Can you work these out from the model? Positions are in its coordinate system, mm. A direction names the side the tool comes from. Coordinates: 2 decimals unless noted, no trailing zeros. Order: outer loops, then holes, each group sorted by start corner. A loop starts at its lowest first (then second) coordinate and runs counter-clockwise, first axis right, second up. Notation, with made-up numbers: (-39.5, -28.75) -> (-3.5, -28.75) arc R31 cw to (-3.5, 10.25) -> close; hole circle Ø10 at (81, -0.75). An arc over 180 degrees is marked (long way). Write item = value, one per line.
```python
from build123d import *

# Parameters (mm, degrees)
BOSS_EXTRUDE1_DEPTH = 3
SKETCH3_OUTSIDE_W   = 181.071
SKETCH3_OUTSIDE_H   = 249.846
SKETCH3_OUTSIDE_W_2 = 131.224989992
SKETCH3_OUTSIDE_H_2 = 70
CUT_EXTRUDE2_DEPTH  = 10
CUT_EXTRUDE3_REACH  = 111.7
SKETCH4_R           = 1.5
CUT_EXTRUDE4_REACH  = 111.7
SKETCH5_W           = 48.153954936
SKETCH5_H           = 90
CUT_EXTRUDE5_REACH  = 111.7
SKETCH6_W           = 16.692706212
SKETCH6_H           = 90.485388772
FILLET1_R           = 10
CUT_EXTRUDE6_REACH  = 102.045
SKETCH8_W           = 12
SKETCH8_H           = 3


with BuildPart() as part:
    # Sketch1 → Boss-Extrude1 (new body)
    with BuildSketch(Plane.XY):
        with BuildLine():
            Line((31.224989992, -95), (31.224989992, 95))
            ThreePointArc((31.224989992, 95), (-100, 0), (31.224989992, -95))
        make_face()
    extrude(amount=BOSS_EXTRUDE1_DEPTH)

    # Sketch3 outside → Cut-Extrude2 (cut)
    with BuildSketch(Plane.XY.offset(3)):
        with Locations((-34.3875, 0)):
            Rectangle(SKETCH3_OUTSIDE_W, SKETCH3_OUTSIDE_H)
        with Locations((-34.387505004, 10)):
            Rectangle(SKETCH3_OUTSIDE_W_2, SKETCH3_OUTSIDE_H_2, mode=Mode.SUBTRACT)
    extrude(amount=-CUT_EXTRUDE2_DEPTH, mode=Mode.SUBTRACT)

    # Sketch4 → Cut-Extrude3 (cut, up to next)
    with BuildSketch(Plane.XY.offset(3), mode=Mode.PRIVATE) as cut_extrude3_sk1:
        with Locations((0, 7)):
            Circle(SKETCH4_R)
    cut_extrude3_tool1 = extrude(cut_extrude3_sk1.sketch, amount=-CUT_EXTRUDE3_REACH, mode=Mode.PRIVATE) & part.part
    # Sketch4 → Cut-Extrude3 (cut, up to next)
    with BuildSketch(Plane.XY.offset(3), mode=Mode.PRIVATE) as cut_extrude3_sk2:
        with Locations((0, -7)):
            Circle(SKETCH4_R)
    cut_extrude3_tool2 = extrude(cut_extrude3_sk2.sketch, amount=-CUT_EXTRUDE3_REACH, mode=Mode.PRIVATE) & part.part
    # Sketch4 → Cut-Extrude3 (cut, up to next)
    with BuildSketch(Plane.XY.offset(3), mode=Mode.PRIVATE) as cut_extrude3_sk3:
        with Locations((7, 0)):
            Circle(SKETCH4_R)
    cut_extrude3_tool3 = extrude(cut_extrude3_sk3.sketch, amount=-CUT_EXTRUDE3_REACH, mode=Mode.PRIVATE) & part.part
    # Sketch4 → Cut-Extrude3 (cut, up to next)
    with BuildSketch(Plane.XY.offset(3), mode=Mode.PRIVATE) as cut_extrude3_sk4:
        with Locations((-7, 0)):
            Circle(SKETCH4_R)
    cut_extrude3_tool4 = extrude(cut_extrude3_sk4.sketch, amount=-CUT_EXTRUDE3_REACH, mode=Mode.PRIVATE) & part.part
    # Sketch4 → Cut-Extrude3 (cut, up to next)
    with BuildSketch(Plane.XY.offset(3), mode=Mode.PRIVATE) as cut_extrude3_sk5:
        Circle(SKETCH4_R)
    cut_extrude3_tool5 = extrude(cut_extrude3_sk5.sketch, amount=-CUT_EXTRUDE3_REACH, mode=Mode.PRIVATE) & part.part
    # Sketch4 → Cut-Extrude3 (cut, up to next)
    with BuildSketch(Plane.XY.offset(3), mode=Mode.PRIVATE) as cut_extrude3_sk6:
        with Locations((0, -21)):
            Circle(SKETCH4_R)
    cut_extrude3_tool6 = extrude(cut_extrude3_sk6.sketch, amount=-CUT_EXTRUDE3_REACH, mode=Mode.PRIVATE) & part.part
    add(cut_extrude3_tool1.solids().sort_by_distance((0, 7, 3))[0], mode=Mode.SUBTRACT)
    add(cut_extrude3_tool2.solids().sort_by_distance((0, -7, 3))[0], mode=Mode.SUBTRACT)
    add(cut_extrude3_tool3.solids().sort_by_distance((7, 0, 3))[0], mode=Mode.SUBTRACT)
    add(cut_extrude3_tool4.solids().sort_by_distance((-7, 0, 3))[0], mode=Mode.SUBTRACT)
    add(cut_extrude3_tool5.solids().sort_by_distance((0, 0, 3))[0], mode=Mode.SUBTRACT)
    add(cut_extrude3_tool6.solids().sort_by_distance((0, -21, 3))[0], mode=Mode.SUBTRACT)

    # Sketch5 → Cut-Extrude4 (cut, up to next)
    with BuildSketch(Plane.XY.offset(3), mode=Mode.PRIVATE) as cut_extrude4_sk1:
        with Locations((36.913108842, 0)):
            Rectangle(SKETCH5_W, SKETCH5_H)
    cut_extrude4_tool1 = extrude(cut_extrude4_sk1.sketch, amount=-CUT_EXTRUDE4_REACH, mode=Mode.PRIVATE) & part.part
    add(cut_extrude4_tool1.solids().sort_by_distance((36.913109, 0, 3))[0], mode=Mode.SUBTRACT)

    # Sketch6 → Cut-Extrude5 (cut, up to next)
    with BuildSketch(Plane.XY.offset(3), mode=Mode.PRIVATE) as cut_extrude5_sk1:
        with Locations((-97.649208603, -0.242694386)):
            Rectangle(SKETCH6_W, SKETCH6_H)
    cut_extrude5_tool1 = extrude(cut_extrude5_sk1.sketch, amount=-CUT_EXTRUDE5_REACH, mode=Mode.PRIVATE) & part.part
    add(cut_extrude5_tool1.solids().sort_by_distance((-97.649209, -0.242694, 3))[0], mode=Mode.SUBTRACT)

    # Fillet1
    fillet1_edges = [part.edges().sort_by_distance(p)[0] for p in [
        (-89.302855497, 45, 1.5),
        (12.836131374, -25, 1.5),
        (12.836131374, 45, 1.5),
        (-89.302855497, -25, 1.5),
    ]]
    fillet(fillet1_edges, radius=FILLET1_R)

    # Sketch8 → Cut-Extrude6 (cut, up to next)
    with BuildSketch(Plane.XY.offset(3), mode=Mode.PRIVATE) as cut_extrude6_sk1:
        with Locations((-72.023868626, 42.359338222)):
            Rectangle(SKETCH8_W, SKETCH8_H)
    cut_extrude6_tool1 = extrude(cut_extrude6_sk1.sketch, amount=-CUT_EXTRUDE6_REACH, mode=Mode.PRIVATE) & part.part
    # Sketch8 → Cut-Extrude6 (cut, up to next)
    with BuildSketch(Plane.XY.offset(3), mode=Mode.PRIVATE) as cut_extrude6_sk2:
        with Locations((-72.023868626, 20.859338222)):
            Rectangle(SKETCH8_W, SKETCH8_H)
    cut_extrude6_tool2 = extrude(cut_extrude6_sk2.sketch, amount=-CUT_EXTRUDE6_REACH, mode=Mode.PRIVATE) & part.part
    add(cut_extrude6_tool1.solids().sort_by_distance((-72.023869, 42.359338, 3))[0], mode=Mode.SUBTRACT)
    add(cut_extrude6_tool2.solids().sort_by_distance((-72.023869, 20.859338, 3))[0], mode=Mode.SUBTRACT)


solid = part.part
```
Item 1: I want a section at C-C, the plane x = -7. Please give me the cut outline in (y, z).
A:
outline = (-25, 0) -> (-1.5, 0) -> (-1.5, 3) -> (-25, 3) -> close; (1.5, 0) -> (45, 0) -> (45, 3) -> (1.5, 3) -> close
Item 2: I'm going to push a flat-ended pin straight in: P1, Ø1.8, axis at x = 0, y = 0, coming from the +Z side. Where does the tip first touch, or does it pass through?
A:
P1 = through
Item 3: I want a section at B-B, the plane z = 1.7. Give the number of separate pieces and of enclosed holes in the cut face, plus the area to 3 significant figures.
A:
separate_pieces = 1
enclosed_holes = 8
area = 6,950 mm2
Item 4: I want a section at D-D, the plane y = 0. Please give me the cut outline in (x, z).
A:
outline = (-89.3, 0) -> (-8.5, 0) -> (-8.5, 3) -> (-89.3, 3) -> close; (-5.5, 0) -> (-1.5, 0) -> (-1.5, 3) -> (-5.5, 3) -> close; (1.5, 0) -> (5.5, 0) -> (5.5, 3) -> (1.5, 3) -> close; (8.5, 0) -> (12.84, 0) -> (12.84, 3) -> (8.5, 3) -> close
Item 5: If I drill on probe 1 along Y at (x, z) = (0, 0.75); probe 2 along Y at (x, z) = (0.5, 2.8); probe 3 along X at (y, z) = (35.5, 2.2), over which ranges is the centre line in solid material (lowest first)?
A:
probe_1 = -25 to -22.5, -19.5 to -8.5, -5.5 to -1.5, 1.5 to 5.5, 8.5 to 45
probe_2 = -25 to -22.41, -19.59 to -8.41, -5.59 to -1.41, 1.41 to 5.59, 8.41 to 45
probe_3 = -89.29 to 12.82
Item 6: I want a section at A-A, the plane y = -7. Please give me the cut outline in (x, z), plus the area to 3 significant figures.
A:
outline = (-89.3, 0) -> (-1.5, 0) -> (-1.5, 3) -> (-89.3, 3) -> close; (1.5, 0) -> (12.84, 0) -> (12.84, 3) -> (1.5, 3) -> close
area = 297 mm2
Item 7: If we mould it in two halves opening along Y, with no side actions, what happens to faces 3 (the flat face through (-89.303, 10, 2)), 4 (the flat face through (-72, 19.359, 2)), 5 (the flat face through (-72, 43.859, 2)), 6 (the cylindrical face through (9.83, 42.15, 1.48))? For each: pulls with the +Y half, pulls with the -Y half, needs draft (parallel to the pull), parting line crosses it, or undercut.
A:
face_3 = needs draft
face_4 = undercut
face_5 = undercut
face_6 = pulls with the +Y half
Item 8: For faces 1 (the flat face through (-72, 22.359, 2)), 2 (the flat face through (12.836, 10, 2)), which set-ups out of +Z, -Z, +X, -X, +Y, -Y let a thin tool reach every point of the face, with its end or its side?
A:
face_1 = +Z, -Z
face_2 = +Z, -Z, +X, +Y, -Y
